```python
from build123d import *

# Parameters (mm, degrees)
SKETCH_1_R          = 15
EXTRUDE_1_DEPTH     = 2.25
SKETCH_2_R          = 4.1
EXTRUDE_2_DEPTH     = 1.4
CHAMFER_1_SIZE      = 1
SKETCH_3_R          = 6.65
EXTRUDE_3_DEPTH     = 3.3
CHAMFER_2_SIZE      = 2.9
CUT_EXTRUDE_2_DEPTH = 3
SKETCH_5_R          = 1.877591738
CUT_EXTRUDE_3_DEPTH = 1
SKETCH_6_R          = 0.7349705
CUT_EXTRUDE_4_DEPTH = 10
SKETCH_7_R          = 1.5
CUT_EXTRUDE_5_DEPTH = 10


with BuildPart() as part:
    # Эскиз1 → Бобышка-Вытянуть1 (new body)
    with BuildSketch(Plane(origin=(0, 0, 0), x_dir=(1, 0, 0), z_dir=(0, 1, 0))):
        with Locations(Location((0, 0, 0), (0, 0, 270))):
            Circle(SKETCH_1_R)
    extrude(amount=EXTRUDE_1_DEPTH)

    # Эскиз2 → Бобышка-Вытянуть2 (add)
    with BuildSketch(Plane(origin=(0, 2.25, 0), x_dir=(1, 0, 0), z_dir=(0, 1, 0))):
        with Locations(Location((0, 0, 0), (0, 0, 270))):
            Circle(SKETCH_2_R)
    extrude(amount=EXTRUDE_2_DEPTH)

    # Фаска1
    chamfer_1_edges = [part.edges().sort_by_distance(p)[0] for p in [
        (0, 3.65, -4.1),
    ]]
    chamfer(chamfer_1_edges, length=CHAMFER_1_SIZE)

    # Эскиз3 → Бобышка-Вытянуть3 (add)
    with BuildSketch(Plane.XZ):
        with Locations(Location((0, 0, 0), (0, 0, 90))):
            Circle(SKETCH_3_R)
    extrude(amount=EXTRUDE_3_DEPTH)

    # Фаска2
    chamfer_2_edges = [part.edges().sort_by_distance(p)[0] for p in [
        (0, -3.3, -6.65),
    ]]
    chamfer(chamfer_2_edges, length=CHAMFER_2_SIZE)

    # Эскиз4 → Вырез-Вытянуть2 (cut)
    with BuildSketch(Plane.XZ.offset(3.3)):
        Polygon((-0.805649398, 2.434445177), (-1.782131202, 1.843801142), (-2.405640065, 0.887969677), (-2.55268241, -0.243735072), (-2.194134697, -1.3271651), (-1.401011698, -2.147733805), (-0.33040115, -2.542917488), (0.805649398, -2.434445177), (1.782131202, -1.843801142), (2.405640065, -0.887969677), (2.55268241, 0.243735072), (2.194134697, 1.3271651), (1.401011698, 2.147733805), (0.33040115, 2.542917488), align=None)
    extrude(amount=-CUT_EXTRUDE_2_DEPTH, mode=Mode.SUBTRACT)

    # Эскиз5 → Вырез-Вытянуть3 (cut)
    with BuildSketch(Plane(origin=(0, 3.65, 0), x_dir=(1, 0, 0), z_dir=(0, 1, 0))):
        with Locations(Location((0, 0, 0), (0, 0, 270))):
            Circle(SKETCH_5_R)
    extrude(amount=-CUT_EXTRUDE_3_DEPTH, mode=Mode.SUBTRACT)

    # Эскиз6 → Вырез-Вытянуть4 (cut)
    with BuildSketch(Plane(origin=(0, 2.65, 0), x_dir=(1, 0, 0), z_dir=(0, 1, 0))):
        with Locations(Location((0, 0, 0), (0, 0, 270))):
            Circle(SKETCH_6_R)
    extrude(amount=-CUT_EXTRUDE_4_DEPTH, mode=Mode.SUBTRACT)

    # Эскиз7 → Вырез-Вытянуть5 (cut)
    with BuildSketch(Plane.XZ):
        with Locations(Location((-7.361215932, -4.25, 0), (0, 0, 270))):
            Circle(SKETCH_7_R)
        with Locations(Location((7.361215932, -4.25, 0), (0, 0, 270))):
            Circle(SKETCH_7_R)
        with Locations(Location((0, 8.5, 0), (0, 0, 270))):
            Circle(SKETCH_7_R)
    extrude(amount=-CUT_EXTRUDE_5_DEPTH, mode=Mode.SUBTRACT)


solid = part.part
```
Read the model definition and answer for the solid it produces. Units are mm, in the model's axes. A direction names the side the tool comes from. Give positions to 0.01 mm unless a question says otherwise; leave off trailing zeros. Order: outer loops, then holes, each group sorted by start corner. A loop starts at its lowest first (then second) coordinate and runs counter-clockwise, first axis right, second up.
(1) Find section B-B (z = 7.75). Give the vertices of the cut face in (x, y), plus the area to 3 significant figures.
(2) Find section A-A (y = -1.75). Give the vertices of the cut face in (x, z), plus the area to 3 significant figures.
(3) Straight lines are drawn through the part: L1, parallel to Z at x = -0.5, y = 1; L2, parallel to X at y = 1.2, z = -4.25; L3, parallel to Z at x = -7.25, y = 2. For each, find the intervals that lie inside material, in ascending order.
(4) Find section D-D (x = 11). Give the vertices of the cut face in (y, z), plus the area to 3 significant figures.
(5) Given pin 1 (1.5 mm diameter, centred on x = 1, z = 0, fed in from +Y); pin 2 (1.5 mm diameter, centred on x = -12, z = 6.5, fed in from -Y); pin 3 (1.5 mm diameter, centred on y = 0.5, z = -9.5, fed in from +X); pin 4 (2.5 mm diameter, centred on x = 0, z = 8.5, fed in from +Y), each flat-ended and moving along its own axis, determine where each tip first touches the part or whether it passes through.
(6) For faces 1 (the flat face through (-0.873, -1.821, -2.343)), 2 (the flat face through (-3, -3.3, 0)), 3 (the cylindrical face through (-1.14, 3.16, -1.49)), determine the directions among +Z, -Z, +X, -X, +Y, -Y from which every point of the face is accessible in a straight line to the end or side of a thin tool.
(7) Find section C-C (y = 1.5). Give the vertices of the cut face in (x, z), plus the area to 3 significant figures.
(8) For a pull along X with two mould halves and no side action, classify faces 4 (the cylindrical face through (4.065, 2.447, -0.534)), 5 (the flat face through (-3.1, 2.25, 3.1)), 6 (the flat face through (1.803, -1.821, 1.732)) as released by +X, released by -X, zero draft, split by the parting line, or undercut.
Result sheet:
1. outline: (-12.84, 0) - (-1.3, 0) - (-1.3, 2.25) - (-12.84, 2.25) - close; (1.3, 0) - (12.84, 0) - (12.84, 2.25) - (1.3, 2.25) - close
1. area: 51.9 mm2
2. outline: circle Ø10.6 at (0, 0); hole (-2.55, -0.24) - (-2.19, -1.33) - (-1.4, -2.15) - (-0.33, -2.54) - (0.81, -2.43) - (1.78, -1.84) - (2.41, -0.89) - (2.55, 0.24) - (2.19, 1.33) - (1.4, 2.15) - (0.33, 2.54) - (-0.81, 2.43) - (-1.78, 1.84) - (-2.41, 0.89) - close
2. area: 68.3 mm2
3. L1: z = -14.99 to -0.54, 0.54 to 7.09, 9.91 to 14.99
3. L2: x = -14.39 to -8.86, -5.86 to 5.86, 8.86 to 14.39
3. L3: z = -13.13 to -5.75, -2.75 to 13.13
4. outline: (0, -10.2) - (2.25, -10.2) - (2.25, 10.2) - (0, 10.2) - close
4. area: 45.9 mm2
5. pin 1: stops at y = 2.65
5. pin 2: stops at y = 0
5. pin 3: stops at x = 12.18
5. pin 4: passes through
6. face 1: -Y
6. face 2: +Z, -Z, +X, -X, -Y
6. face 3: +Y
7. outline: circle Ø30 at (0, 0); hole circle Ø3 at (-7.36, -4.25); hole circle Ø3 at (0, 8.5); hole circle Ø1.47 at (0, 0); hole circle Ø3 at (7.36, -4.25)
7. area: 684 mm2
8. face 4: split by the parting line
8. face 5: zero draft
8. face 6: undercut
